Check sheet for the drawn part. Datum: minimum x, y, z corner. Units: mm. A direction names the side the tool comes from. Round coordinates to 2 decimals unless told otherwise and drop trailing zeros. Write each loop counter-clockwise with the first axis right and the second up, starting at its lowest first coordinate (ties: lowest second). Pieces come first, ordered by that corner, then holes. Notation, with made-up numbers: M -32,82 L -21,82 A13 cw -21,98 Z; hole C 30.5,52 d9. An arc over 180 degrees is marked long. One line per item, written item: value. Start each with the question number.
Item 1: Thickness scan on probe 1 along X at (y, z) = (13.75, 7.5); probe 2 along Y at (x, z) = (5.5, 1.75); probe 3 along X at (y, z) = (10.25, 10.75). Record the ranges inside material, lowest first. Write a range as from..to.
Item 2: Section check A-A, the plane y = 10. State how many separate pieces and enclosed holes the cut face has.
Item 3: Section check D-D, the plane x = 1.75. Record the cut outline in (y, z), then the cut area to 3 significant figures.
Item 4: Section check C-C, the plane z = 6.5. Record the cut outline in (x, y) (1 decimal).
Item 5: Tool access check on the marked faces 1, 2, 3 and 4. Record the directions out of +Z, -Z, +X, -X, +Y, -Y that give a thin tool (end or side, any length) a straight path to the whole face; none if there is none.
Item 6: Draft check along Y on the marked faces 5, 6 and 7. Enter one of: +Y half, -Y half, draft (parallel to the pull), parting line (faces both ways), or undercut.
Item 7: Gauge pin test, flat ends, axial feed: pin 1 (5 mm diameter, centred on y = 8.5, z = 5.5, fed in from +X); pin 2 (12 mm diameter, centred on x = 17.5, z = 13, fed in from +Y); pin 3 (1 mm diameter, centred on x = 8, y = 8, fed in from -Z); pin 4 (10 mm diameter, centred on x = 10, y = 10, fed in from +Z). Record the tip position at first contact, or that the pin passes through.
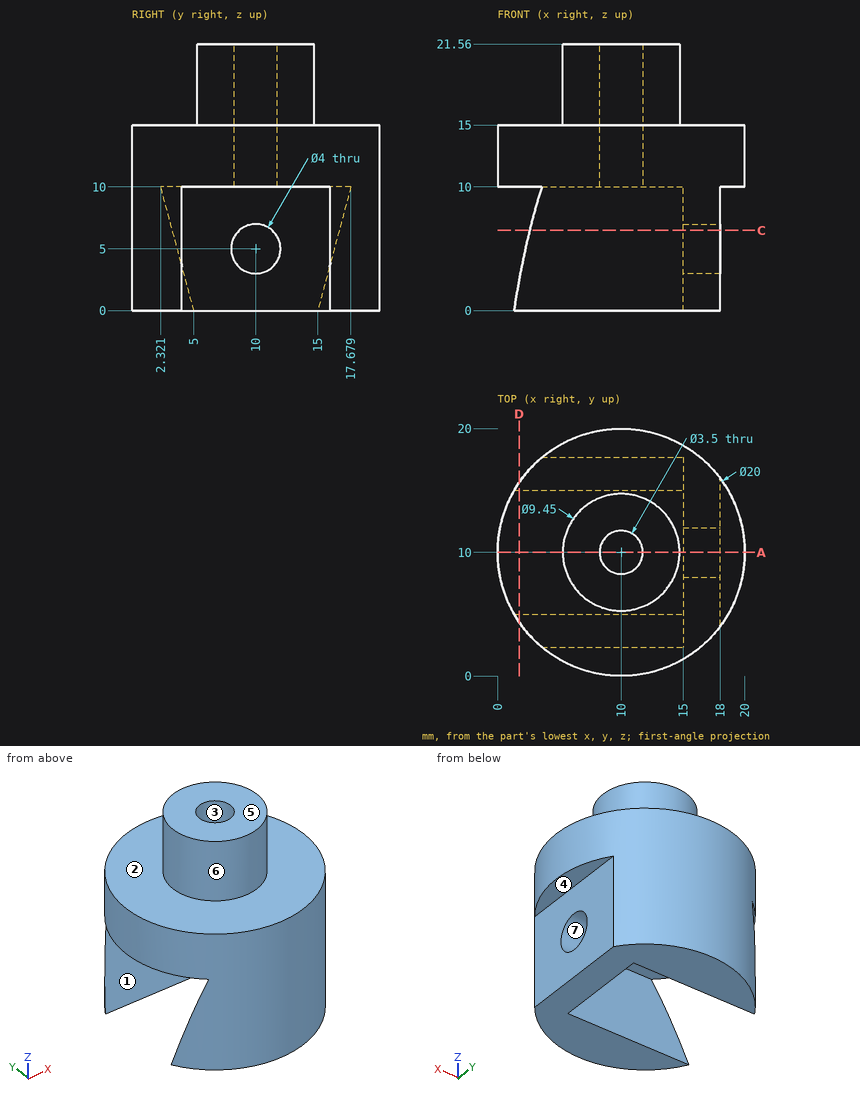
Response values:
1. probe 1: x = 15..18
1. probe 2: y = 1.07..4.53, 15.47..18.93
1. probe 3: x = 0..8.27, 11.73..20
2. separate pieces: 3
2. enclosed holes: 0
3. outline: M 4.35,0 L 5,0 L 4.35,2.43 Z; M 4.35,10 L 15.65,10 L 15.65,15 L 4.35,15 Z; M 15,0 L 15.65,0 L 15.65,2.43 Z
3. area: 58.1 mm2
4. outline: M 2.6,3.3 A10 ccw 18,4 L 18,8.7 L 15,8.7 L 15,3.3 Z; M 2.6,16.7 L 15,16.7 L 15,11.3 L 18,11.3 L 18,16 A10 ccw Z
5. face 1: -X
5. face 2: +Z
5. face 3: +Z, -Z
5. face 4: -Z, +X, +Y, -Y
6. face 5: draft
6. face 6: parting line
6. face 7: undercut
7. pin 1: stops at x = 18
7. pin 2: stops at y = 19.89
7. pin 3: stops at z = 10
7. pin 4: stops at z = 21.56
